Check sheet for the drawn part. Datum: minimum x, y, z corner. Units: mm. Give positions to 0.01 mm unless a question says otherwise; leave off trailing zeros. Loops run counter-clockwise (first coordinate to the right, second up) from the corner with the lowest first, then second, coordinate; pieces in that order, holes last. Notation, with made-up numbers: (-38.75, -30.5) - (-18.75, -30.5) arc R25 cw to (-18.75, 6.5) - close; hole circle Ø8 at (15, 28). An arc over 180 degrees is marked (long way). One line per item, written item: value. Start each with the question number.
1. Sectioned sample at B-B (z = 7.5). Record the cut outline in (x, y).
2. Sectioned sample at C-C (x = 20.5). Record the cut outline in (y, z).
3. Gauge pin test, flat ends, axial feed: pin 1 (1 mm diameter, centred on x = 10.5, y = 7, fed in from +Z); pin 2 (1 mm diameter, centred on y = 14, z = 3, fed in from -X); pin 3 (1.6 mm diameter, centred on y = 17.5, z = 7, fed in from -X). Record the tip position at first contact, or that the pin passes through.
4. Sectioned sample at D-D (y = 25). Record the cut outline in (x, z), plus the area to 3 significant figures.
5. Sectioned sample at A-A (z = 4). Record the cut outline in (x, y), plus the area to 3 significant figures.
6. Mould release check, pull along X, two halves, no side actions. Record for the marked faces 1, 2 and 3: pulls with the +X half, pulls with the -X half, needs draft (parallel to the pull), parting line crosses it, or undercut.
7. Scan lines: L1, parallel to X at y = 16, z = 5.5; L2, parallel to Y at x = 28, z = 7.25; L3, parallel to X at y = 31.5, z = 6.5. Record each from-to range of solid material in increasing order. Write a range as [from, to].
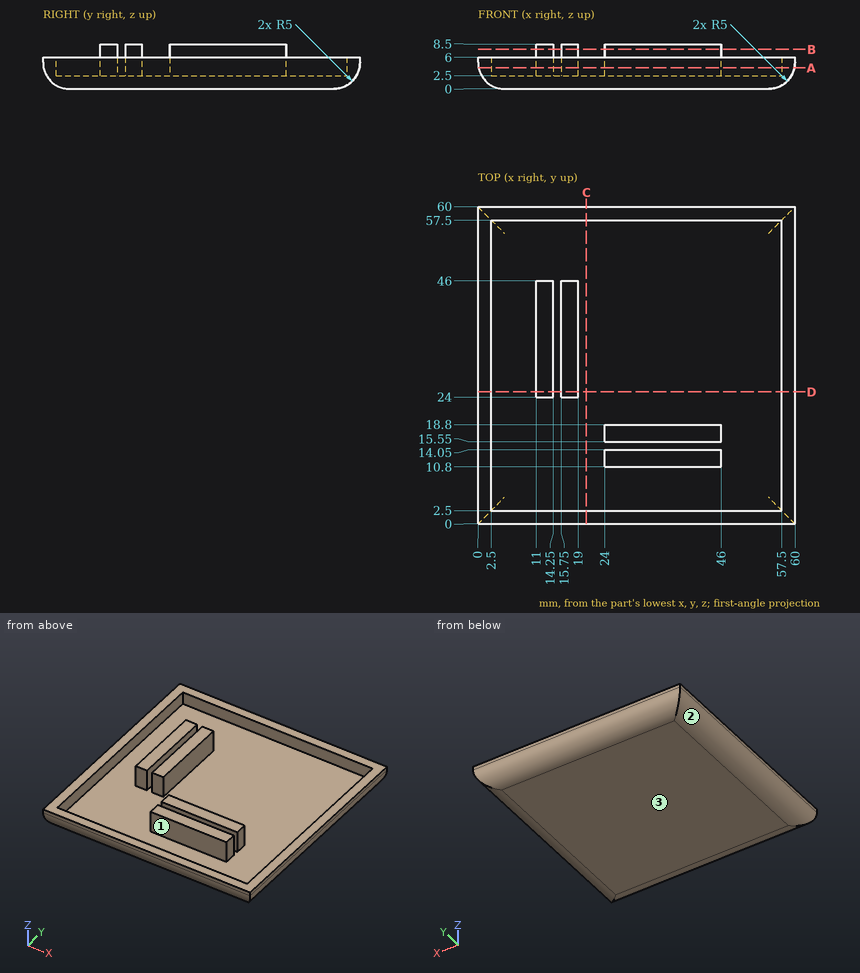
Results are:
1. outline: (11, 24) - (14.25, 24) - (14.25, 46) - (11, 46) - close; (15.75, 24) - (19, 24) - (19, 46) - (15.75, 46) - close; (24, 10.8) - (46, 10.8) - (46, 14.05) - (24, 14.05) - close; (24, 15.55) - (46, 15.55) - (46, 18.8) - (24, 18.8) - close
2. outline: (0, 5) arc R5 ccw to (5, 0) - (55, 0) arc R5 ccw to (60, 5) - (60, 6) - (57.5, 6) - (57.5, 2.5) - (2.5, 2.5) - (2.5, 6) - (0, 6) - close
3. pin 1: stops at z = 2.5
3. pin 2: stops at x = 0.23
3. pin 3: stops at x = 24
4. outline: (0, 5) arc R5 ccw to (5, 0) - (55, 0) arc R5 ccw to (60, 5) - (60, 6) - (57.5, 6) - (57.5, 2.5) - (19, 2.5) - (19, 8.5) - (15.75, 8.5) - (15.75, 2.5) - (14.25, 2.5) - (14.25, 8.5) - (11, 8.5) - (11, 2.5) - (2.5, 2.5) - (2.5, 6) - (0, 6) - close
4. area: 196 mm^2
5. outline: (0.1, 0.1) - (59.9, 0.1) - (59.9, 59.9) - (0.1, 59.9) - close; (11, 24) - (14.25, 24) - (14.25, 46) - (11, 46) - close; (15.75, 24) - (19, 24) - (19, 46) - (15.75, 46) - close; (24, 10.8) - (46, 10.8) - (46, 14.05) - (24, 14.05) - close; (24, 15.55) - (46, 15.55) - (46, 18.8) - (24, 18.8) - close; hole (2.5, 2.5) - (57.5, 2.5) - (57.5, 57.5) - (2.5, 57.5) - close
5. area: 837 mm^2
6. face 1: undercut
6. face 2: pulls with the -X half
6. face 3: needs draft
7. L1: x = [0, 2.5], [24, 46], [57.5, 60]
7. L2: y = [10.8, 14.05], [15.55, 18.8]
7. L3: x = [11, 14.25], [15.75, 19]
